Check sheet for the modelled part. Datum: model origin and axes. Units: mm. Face numbers are marked on the shaded views. A direction names the side the tool comes from. Give positions to 0.01 mm unless a question says otherwise; leave off trailing zeros. Loops run counter-clockwise (first coordinate to the right, second up) from the corner with the lowest first, then second, coordinate; pieces in that order, holes last. Notation, with made-up numbers: M -23.5,85.25 L 25.5,85.25 A15 ccw 25.5,102.25 Z; hole C 71,-6.75 d1. An arc over 180 degrees is marked long. Write each question's results on one line, items separated by ' | '. Start each with the question number.
1. Sectioned sample at C-C on y = 4.5. Record the cut outline in (x, z), and give its area (3 significant figures).
2. Go/stop test with flat-tipped pins: pin 1 (0.8 mm diameter, centred on x = 4.5, y = 2.5, fed in from -Z); pin 2 (9 mm diameter, centred on x = 6.5, y = 5.5, fed in from +Z); pin 3 (3 mm diameter, centred on x = 4.5, z = 1.5, fed in from +Y). Record where each tip stops, or that it passes through.
3. Tool access check on the marked faces 4 and 5. Record the directions out of +Z, -Z, +X, -X, +Y, -Y that give a thin tool (end or side, any length) a straight path to the whole face; none if there is none.
4. Material ranges on line 1 along Y through (x, z) = (4.75, 1); line 2 along Y through (x, z) = (4.5, 0.9); line 3 along X through (y, z) = (2.5, 0.95), recorded low to high.
5. Sectioned sample at A-A on x = 14. Record the cut outline in (y, z), and give its area (3 significant figures).
6. Sectioned sample at D-D on y = -0.25. Record the cut outline in (x, z), and give its area (3 significant figures).
7. Sectioned sample at B-B on z = 0.95. Record the cut outline in (x, y), and give its area (3 significant figures).
8. Draft check along X on the marked faces 1, 2 and 3. Enter one of: pulls with the +X half, pulls with the -X half, needs draft (parallel to the pull), parting line crosses it, or undercut.
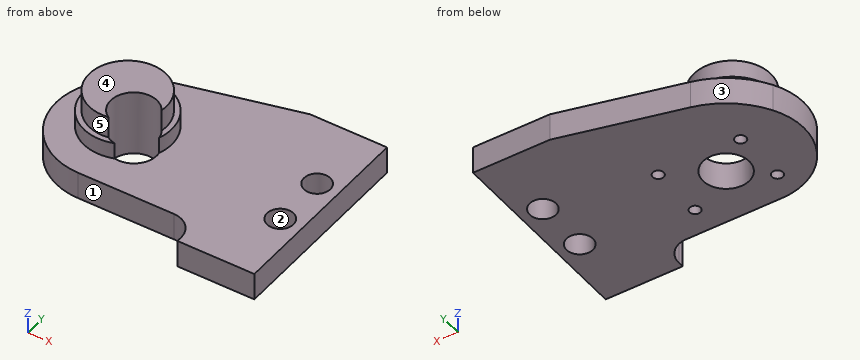
Autodesk Inventor part; units mm, degrees
ref_plane "YZ Plane" through (0, 0, 0) normal (1, 0, 0) x (0, 1, 0)
ref_plane "XZ Plane" through (0, 0, 0) normal (0, 1, 0) x (-1, 0, 0)
ref_plane "XY Plane" through (0, 0, 0) normal (0, 0, 1) x (1, 0, 0)
sketch "MCP joint" plane through (0, 0, 0) normal (0, 0, 1) x (1, 0, 0)
  point P0 (0, 0)
  point P1 (0, 0)
sketch "Sketch2" plane through (0, 0, 0) normal (0, 0, 1) x (1, 0, 0)
  line L0 (9, -7.5) -> (16, -7.5)
  line L1 (16, -7.5) -> (16, 10.5)
  line L2 (16, 10.5) -> (9, 10.5)
  circle A0 centre (0, 0) radius 8
  line L3 (9, 10.5) -> (-1.9428, 7.7605)
  line L4 (9, -7.5) -> (0.4552, -7.987)
  point P0 (16, 1.5)
  point P1 (3.5, 1.5)
  point P2 (16, 1.5)
  dimension "d0" = 18
  dimension "d3" = 16
  dimension "d94" = 1.5
  dimension "d95" = 16
  dimension "d96" = 9
  dimension "d97" = 9
extrude "base" add sketch "Sketch2" along normal blind 2.5
sketch "Sketch3" plane through (0, 0, 2.5) normal (0, 0, 1) x (1, 0, 0)
  point P0 (0, 0)
  point P1 (0, 0)
hole "bearing pocket" at (0, 0, 2.5) direction (0, 0, -1) diameter 4 end through all
sketch "Sketch13" plane through (0, 0, 0) normal (0, 0, -1) x (-1, 0, 0)
  line L0 (-9, -7.5) -> (-9, -5)
  arc A0 (-0.4552, -7.987) -> (1.9428, 7.7605) centre (0, 0) ccw
  line L1 (-9, -5) -> (6.245, -5)
  line L2 (-0.4552, -7.987) -> (-9, -7.5)
  dimension "d76" = 2.5
extrude "bottom cutout" cut sketch "Sketch13" against normal through all
fillet "Fillet2" radius 2 1 edges at (9, -5, 1.25)
fillet "Fillet4" radius 6 1 edges at (-6.245, -5, 1.25)
sketch "Sketch7" plane through (0, 0, 0) normal (0, 0, -1) x (-1, 0, 0)
  line L0 (3, 2.5) -> (-4.5, 2.5) construction
  line L1 (-4.5, 2.5) -> (-4.5, -2.5) construction
  line L2 (-4.5, -2.5) -> (3, -2.5) construction
  line L3 (3, -2.5) -> (3, 2.5) construction
  line L4 (3, 2.5) -> (-4.5, -2.5) construction
  line L5 (-4.5, 2.5) -> (3, -2.5) construction
  point P0 (0, 0)
  point P1 (-0.75, 0)
  point P2 (0, 0)
  point P3 (-0.75, 0)
  dimension "d34" = 3
  dimension "d35" = 4.5
  dimension "d36" = 5
hole "potentiometer pins" at (-3, 2.5, 0) at (-3, -2.5, 0) at (4.5, -2.5, 0) at (4.5, 2.5, 0) direction (0, 0, 1) diameter 1 depth 1.5
sketch "Sketch8" plane through (0, 0, 2.5) normal (0, 0, 1) x (1, 0, 0)
  line L0 (8.1428, 0) -> (0, 0) construction
  line L1 (0, 0) -> (-8.8782, 8.8782) construction
  circle A0 centre (-1.6971, 1.6971) radius 3.5
  dimension "d45" = 2.4
  dimension "d46" = 7
  dimension "d59" = 45
extrude "bearing" add sketch "Sketch8" along normal blind 3.5
sketch "Sketch10" plane through (0, 0, 2.5) normal (0, 0, 1) x (1, 0, 0)
  circle A0 centre (-1.6971, 1.6971) radius 3.5
  circle A1 centre (-1.6971, 1.6971) radius 4
  point P0 (0, 0)
  point P1 (1.0607, -1.0607)
  dimension "d56" = 8
extrude "bearing spacer" add sketch "Sketch10" along normal blind 1.5
sketch "Sketch11" plane through (-1.6971, 1.6971, 6) normal (0, 0, 1) x (1, 0, 0)
  point P0 (1.6971, -1.6971)
  point P1 (1.6971, -1.6971)
hole "Hole4" at (0, 0, 6) direction (0, 0, -1) diameter 4.2 end through all
sketch "Sketch12" plane through (0, 0, 2.5) normal (0, 0, 1) x (1, 0, 0)
  point P0 (0, 0)
  point P1 (14, 4)
  point P2 (14, -1)
  point P3 (0, 0)
  dimension "d88" = 14
  dimension "d89" = 14
  dimension "d90" = 4
  dimension "d91" = 1
hole "mounting" at (14, 4, 2.5) at (14, -1, 2.5) direction (0, 0, -1) diameter 2.4 end through all
equation "\"MCP_spring_arm\" = F4_MCP_spring_arm"
properties part number "MCP mount M F4"
Output values:
1) outline: M -6.61,0 L 12.91,0 L 12.91,2.5 L 1.16,2.5 L 1.16,4 L 0.4,4 L 0.4,6 L -3.79,6 L -3.79,4 L -4.55,4 L -4.55,2.5 L -6.61,2.5 Z; M 15.09,0 L 16,0 L 16,2.5 L 15.09,2.5 Z | area: 68.0 mm2
2) pin 1: z = 1.5 | pin 2: z = 2.5 | pin 3: y = 9.75
3) face 4: +Z, +X, -X, +Y, -Y | face 5: +Z
4) line 1: -5 to -2.93, -2.07 to 2.07, 2.93 to 9.44 | line 2: -5 to -3, -2 to 2, 3 to 9.37 | line 3: -7.54 to -3.5, -2.5 to 4, 5 to 16
5) outline: M -7.5,0 L -2.2,0 L -2.2,2.5 L -7.5,2.5 Z; M 0.2,0 L 2.8,0 L 2.8,2.5 L 0.2,2.5 Z; M 5.2,0 L 10.5,0 L 10.5,2.5 L 5.2,2.5 Z | area: 33.0 mm2
6) outline: M -7.6,0 L -2.09,0 L -2.09,6 L -4.61,6 L -4.61,4 L -5.19,4 L -5.19,2.5 L -7.6,2.5 Z; M 2.09,0 L 13.06,0 L 13.06,2.5 L 2.09,2.5 Z; M 14.94,0 L 16,0 L 16,2.5 L 14.94,2.5 Z | area: 53.6 mm2
7) outline: M -6.93,4 A6 ccw -1.73,-5 L 7,-5 A2 cw 9,-7 L 9,-7.5 L 16,-7.5 L 16,10.5 L 9,10.5 L -1.94,7.76 A8 ccw Z; hole C -3,-2.5 d1; hole C -3,2.5 d1; hole C 0,0 d4.2; hole C 4.5,-2.5 d1; hole C 4.5,2.5 d1; hole C 14,-1 d2.4; hole C 14,4 d2.4 | area: 311 mm2
8) face 1: needs draft | face 2: undercut | face 3: pulls with the -X half
